```python
from build123d import *

# Parameters (mm, degrees)
SKETCH2_W               = 35
SKETCH2_H               = 2
CUT_EXTRUDE1_DEPTH      = 35.223529917
CUT_EXTRUDE1_DEPTH_BACK = 35.223529917
SKETCH3_W               = 14
SKETCH3_H               = 4
CUT_EXTRUDE2_DEPTH      = 35.731109974
CUT_EXTRUDE2_DEPTH_BACK = 35.731109974
SKETCH4_R               = 2


with BuildPart() as part:
    # Sweep1: sweep along a path in Sketch1
    with BuildLine(Plane.XY) as sweep1_path:
        Line((24, -16), (13.25, -16))
        ThreePointArc((13.25, -16), (12.366116524, -15.633883476), (12, -14.75))
        Line((12, -14.75), (12, -1.25))
        ThreePointArc((12, -1.25), (11.633883476, -0.366116524), (10.75, 0))
        Line((10.75, 0), (-10.75, 0))
        ThreePointArc((-10.75, 0), (-11.633883476, -0.366116524), (-12, -1.25))
        Line((-12, -1.25), (-12, -14.75))
        ThreePointArc((-12, -14.75), (-12.366116524, -15.633883476), (-13.25, -16))
        Line((-13.25, -16), (-24, -16))
    # Sketch2 → Sweep1 (sweep)
    with BuildSketch(Plane(origin=(0, 0, 0), x_dir=(0, 0, -1), z_dir=(1, 0, 0))):
        Rectangle(SKETCH2_W, SKETCH2_H)
    sweep(path=sweep1_path.line)

    # Sketch3 → Cut-Extrude1 (cut, two sides: drawn at the far end of the back side and taken through both)
    with BuildSketch(Plane(origin=(0, 0, 0), x_dir=(0, 0, -1), z_dir=(1, 0, 0)).offset(-CUT_EXTRUDE1_DEPTH_BACK)):
        with Locations((-10.5, -1)):
            Rectangle(SKETCH3_W, SKETCH3_H)
    extrude(amount=CUT_EXTRUDE1_DEPTH + CUT_EXTRUDE1_DEPTH_BACK, mode=Mode.SUBTRACT)

    # Sketch4 → Cut-Extrude2 (cut, two sides: drawn at the far end of the back side and taken through both)
    with BuildSketch(Plane(origin=(0, 1, 0), x_dir=(1, 0, 0), z_dir=(0, 1, 0)).offset(-CUT_EXTRUDE2_DEPTH_BACK)):
        with Locations(Location((0, 1.5, 0), (0, 0, 180))):
            Circle(SKETCH4_R)
        with Locations(Location((0, 9.5, 0), (0, 0, 180))):
            Circle(SKETCH4_R)
        with Locations(Location((-19, 12.5, 0), (0, 0, 180))):
            Circle(SKETCH4_R)
        with Locations(Location((-19, -12.5, 0), (0, 0, 180))):
            Circle(SKETCH4_R)
        with Locations(Location((19, -12.5, 0), (0, 0, 180))):
            Circle(SKETCH4_R)
        with Locations(Location((19, 12.5, 0), (0, 0, 180))):
            Circle(SKETCH4_R)
    extrude(amount=CUT_EXTRUDE2_DEPTH + CUT_EXTRUDE2_DEPTH_BACK, mode=Mode.SUBTRACT)


solid = part.part
```
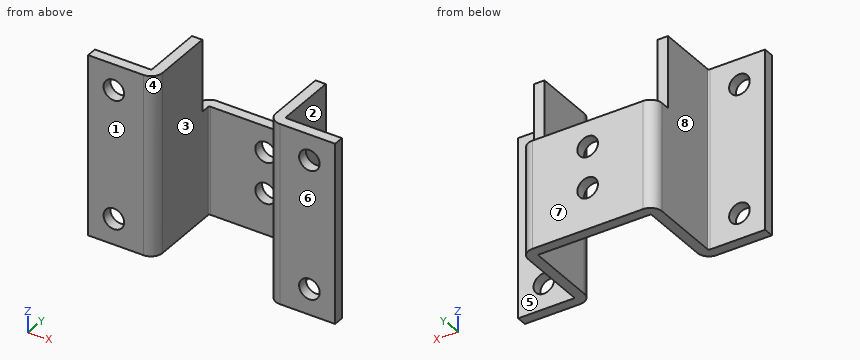
Input: part model. Units: mm. Frame: model coordinates. Face numbers are marked on the shaded views. A direction names the side the tool comes from. Give positions to 0.01 mm unless a question says otherwise; leave off trailing zeros. Order: outer loops, then holes, each group sorted by start corner. A loop starts at its lowest first (then second) coordinate and runs counter-clockwise, first axis right, second up.
1. Set-up query: the marked faces 4, 5, 6, 7 and 8. Return all of +Z, -Z, +X, -X, +Y, -Y with unobstructed straight access to the full face (end or side cutting, diameter ignored); none if empty.
Computed:
face 4: +Z, -Z, -Y
face 5: +Z, -Z, +X, +Y
face 6: +Z, -Z, +X, -X, -Y
face 7: +Z, -Z, +X, -X, +Y
face 8: +Z, -Z, -X, +Y
2. Line query: probe 1 along Z at (x, y) = (19, -15.9); probe 2 along Z at (x, y) = (0, -0.05); probe 3 along X at (y, z) = (-3.75, 13). Output: solid intervals per line, ascending.
Computed:
probe 1: z = -17.5 to -14.5, -10.5 to 10.5, 14.5 to 17.5
probe 2: z = -17.5 to -11.5, -7.5 to -3.5, 0.5 to 3.5
probe 3: x = -13 to -11, 11 to 13
3. Pin query (flat end, axial travel): pin 1 Ø3 at (x, z) = (-21, 6) entering from +Y; pin 2 Ø4 at (y, z) = (-9, 7) entering from -X; pin 3 Ø6 at (x, z) = (11.5, 10) entering from -Y; pin 4 Ø6 at (y, z) = (-10.5, 10.5) entering from +X. Return the tip coordinate at first contact, or that it passes through.
Computed:
pin 1: stops at y = -15
pin 2: stops at x = -13
pin 3: stops at y = -17
pin 4: stops at x = 13
4. Cut plane C-C (x = 19). Return loops of the section in (y, z).
Computed:
outline: (-17, -17.5) - (-15, -17.5) - (-15, -14.5) - (-17, -14.5) - close; (-17, -10.5) - (-15, -10.5) - (-15, 10.5) - (-17, 10.5) - close; (-17, 14.5) - (-15, 14.5) - (-15, 17.5) - (-17, 17.5) - close
5. Cut plane D-D (z = -9.5). Return loops of the section in (x, y).
Computed:
outline: (-24, -17) - (-13.25, -17) arc R2.25 ccw to (-11, -14.75) - (-11, -1.25) arc R0.25 cw to (-10.75, -1) - (-2, -1) - (-2, 1) - (-10.75, 1) arc R2.25 ccw to (-13, -1.25) - (-13, -14.75) arc R0.25 cw to (-13.25, -15) - (-24, -15) - close; (2, -1) - (10.75, -1) arc R0.25 cw to (11, -1.25) - (11, -14.75) arc R2.25 ccw to (13.25, -17) - (24, -17) - (24, -15) - (13.25, -15) arc R0.25 cw to (13, -14.75) - (13, -1.25) arc R2.25 ccw to (10.75, 1) - (2, 1) - close
6. Cut plane B-B (z = 12.5). Return loops of the section in (x, y), and give its area (3 significant figures).
Computed:
outline: (-24, -17) - (-21, -17) - (-21, -15) - (-24, -15) - close; (-17, -17) - (-13.25, -17) arc R2.25 ccw to (-11, -14.75) - (-11, -3) - (-13, -3) - (-13, -14.75) arc R0.25 cw to (-13.25, -15) - (-17, -15) - close; (11, -14.75) arc R2.25 ccw to (13.25, -17) - (17, -17) - (17, -15) - (13.25, -15) arc R0.25 cw to (13, -14.75) - (13, -3) - (11, -3) - close; (21, -17) - (24, -17) - (24, -15) - (21, -15) - close
area: 81.9 mm2
7. Draft query along X for the marked faces 1, 2 and 3. Return one class per face: released by +X, released by -X, zero draft, split by the parting line, or undercut.
Computed:
face 1: zero draft
face 2: released by +X
face 3: undercut
8. Cut plane A-A (y = -1.75). Return loops of the section in (x, z).
Computed:
outline: (-13, -17.5) - (-11, -17.5) - (-11, 3.5) - (-13, 3.5) - close; (11, -17.5) - (13, -17.5) - (13, 3.5) - (11, 3.5) - close
